```python
from build123d import *

# Parameters (mm, degrees)
PAD001_DEPTH    = 22
SKETCH_W        = 44
SKETCH_H        = 5
PAD_DEPTH       = 22
SKETCH001_W     = 20
SKETCH001_H     = 25
POCKET_DEPTH    = 3
SKETCH003_R     = 1.1
POCKET001_DEPTH = 5
SKETCH004_R     = 1.1
POCKET002_DEPTH = 5
SKETCH005_W     = 20
SKETCH005_H     = 7
POCKET003_DEPTH = 2.001
SKETCH007_R     = 2
POCKET004_DEPTH = 3.5


with BuildPart() as pad001:
    # Sketch002 → Pad001 (new body, symmetric)
    with BuildSketch(Plane.YZ):
        with BuildLine():
            Line((-22, 0), (22, 0))
            Line((22, 0), (22, 2))
            ThreePointArc((22, 2), (0, 5), (-22, 2))
            Line((-22, 2), (-22, 0))
        make_face()
    extrude(amount=PAD001_DEPTH, both=True)


with BuildPart() as obj1:
    # Sketch → Pad (new body, symmetric)
    with BuildSketch(Plane.XZ):
        with Locations((0, 2.5)):
            Rectangle(SKETCH_W, SKETCH_H)
    extrude(amount=PAD_DEPTH, both=True)

    # Sketch001 → Pocket (cut)
    with BuildSketch(Plane(origin=(0, 0, 5), x_dir=(-1, 0, 0), z_dir=(0, 0, 1))):
        Rectangle(SKETCH001_W, SKETCH001_H)
    extrude(amount=-POCKET_DEPTH, mode=Mode.SUBTRACT)

    # Common: intersect Pad001
    add(pad001.part, mode=Mode.INTERSECT)

    # Sketch003 → Pocket001 (cut)
    with BuildSketch(Plane.YZ.offset(-10)):
        with Locations((6.5, 3.3)):
            Circle(SKETCH003_R)
    extrude(amount=-POCKET001_DEPTH, mode=Mode.SUBTRACT)

    # Sketch004 → Pocket002 (cut)
    with BuildSketch(Plane(origin=(10, 0, 0), x_dir=(0, -1, 0), z_dir=(-1, 0, 0))):
        with Locations((-6.5, 3.3)):
            Circle(SKETCH004_R)
    extrude(amount=-POCKET002_DEPTH, mode=Mode.SUBTRACT)

    # Sketch005 → Pocket003 (cut, through all)
    with BuildSketch(Plane.XY.offset(2)):
        with Locations((0, 9)):
            Rectangle(SKETCH005_W, SKETCH005_H)
    extrude(amount=-POCKET003_DEPTH, mode=Mode.SUBTRACT)

    # Sketch007 → Pocket004 (cut)
    with BuildSketch(Plane(origin=(0, 0, 0), x_dir=(1, 0, 0), z_dir=(0, 0, -1))):
        with Locations((-16, 0)):
            Circle(SKETCH007_R)
        with Locations((16, 0)):
            Circle(SKETCH007_R)
    extrude(amount=-POCKET004_DEPTH, mode=Mode.SUBTRACT)


solid = obj1.part
```
Input: part model. Units: mm. Frame: model coordinates. A direction names the side the tool comes from. Give positions to 0.01 mm unless a question says otherwise; leave off trailing zeros. Order: outer loops, then holes, each group sorted by start corner. A loop starts at its lowest first (then second) coordinate and runs counter-clockwise, first axis right, second up. Notation, with made-up numbers: (-23.75, -29) -> (-13.75, -29) arc R24 cw to (-13.75, -8) -> close; hole circle Ø10 at (-4.5, -25). An arc over 180 degrees is marked (long way). Write each question's results on one line, items separated by ' | '. Start each with the question number.
Item 1: Cut plane B-B on z = 1.4. Return the cut outline in (x, y).
Item 2: Set-up query: faces 1 (the flat face through (0, -12.5, 3)), 2 (the cylindrical face through (-17.6, 1.2, 1.7)), 3 (the cylindrical face through (12.465, 5.484, 2.879)). Return all of +Z, -Z, +X, -X, +Y, -Y with unobstructed straight access to the full face (end or side cutting, diameter ignored); none if empty.
Item 3: Contact query for flat-ended pins moving along their axis: P1, Ø1.2, axis at x = -16.5, y = -0.5, coming from the -Z side; P2, Ø20, axis at x = 3, y = -3.5, coming from the +Z side; P3, Ø5, axis at x = -16, y = 12, coming from the +Z side. Output: stop coordinate, or through.
Item 4: Cut plane C-C on y = 0. Return the cut outline in (x, z), then the cut area to 3 significant figures.
Item 5: Cut plane D-D on x = -16. Return the cut outline in (y, z), then the cut area to 3 significant figures.
Item 6: Cut plane A-A on x = -8. Return the cut outline in (y, z), then the cut area to 3 significant figures.
Item 7: Mould query, pull axis X, two halves, no side actions, for faces 4 (the flat face through (-22, 0, 2)), 5 (the flat face through (0, -22, 1)), 6 (the flat face through (0, 5.5, 1)). Classes: pulls with the +X half, pulls with the -X half, needs draft (parallel to the pull), parting line crosses it, or undercut.
Item 8: Line query: line 1 (X direction, y = 0, z = 2.7); line 2 (X direction, y = 0, z = 1.3); line 3 (Y direction, x = -16, z = 0.95). Output: solid intervals per line, ascending.
Established:
1) outline: (-22, -22) -> (22, -22) -> (22, 22) -> (-22, 22) -> close; hole circle Ø4 at (-16, 0); hole (-10, 5.5) -> (10, 5.5) -> (10, 12.5) -> (-10, 12.5) -> close; hole circle Ø4 at (16, 0)
2) face 1: +Z | face 2: -Z | face 3: none
3) P1: z = 3.5 | P2: z = 5 | P3: z = 4.45
4) outline: (-22, 0) -> (-18, 0) -> (-18, 3.5) -> (-14, 3.5) -> (-14, 0) -> (14, 0) -> (14, 3.5) -> (18, 3.5) -> (18, 0) -> (22, 0) -> (22, 5) -> (10, 5) -> (10, 2) -> (-10, 2) -> (-10, 5) -> (-22, 5) -> close | area: 132 mm^2
5) outline: (-22, 0) -> (-2, 0) -> (-2, 3.5) -> (2, 3.5) -> (2, 0) -> (22, 0) -> (22, 2) arc R82.17 ccw to (-22, 2) -> close | area: 162 mm^2
6) outline: (-22, 0) -> (5.5, 0) -> (5.5, 2) -> (-12.5, 2) -> (-12.5, 4.04) arc R82.17 ccw to (-22, 2) -> close; (12.5, 0) -> (22, 0) -> (22, 2) arc R82.17 ccw to (12.5, 4.04) -> close | area: 95.3 mm^2
7) face 4: pulls with the -X half | face 5: needs draft | face 6: undercut
8) line 1: -22 to -18, -14 to -10, 10 to 14, 18 to 22 | line 2: -22 to -18, -14 to 14, 18 to 22 | line 3: -22 to -2, 2 to 22
